Autodesk Inventor part; units mm, degrees
ref_plane "YZ Plane" through (0, 0, 0) normal (1, 0, 0) x (0, 1, 0)
ref_plane "XZ Plane" through (0, 0, 0) normal (0, 1, 0) x (-1, 0, 0)
ref_plane "XY Plane" through (0, 0, 0) normal (0, 0, 1) x (1, 0, 0)
sketch "main" plane through (0, 0, 0) normal (0, 0, 1) x (1, 0, 0)
  circle A0 centre (11.2296, 26.3602) radius 2.1844
  line L0 (23.9296, 20.0102) -> (22.6596, 20.0102)
  line L1 (4.8796, 31.6942) -> (5.8956, 32.7102)
  circle A1 centre (23.9296, 26.3602) radius 2.1844
  line L2 (23.9296, 32.7102) -> (5.8956, 32.7102)
  arc A2 (23.9296, 20.0102) -> (23.9296, 32.7102) centre (23.9296, 26.3602) ccw
  circle A3 centre (-14.1704, -24.4398) radius 2.1844
  circle A4 centre (11.2296, -24.4398) radius 2.1844
  arc A5 (22.6596, 20.0102) -> (4.8796, 2.2302) centre (22.6596, 2.2302) ccw
  line L3 (4.8796, -11.7398) -> (4.8796, 2.2302)
  arc A6 (4.8796, -11.7398) -> (11.2296, -18.0898) centre (11.2296, -11.7398) ccw
  line L4 (4.8796, 31.6942) -> (-20.5204, -19.1058)
  arc A7 (11.2296, -30.7898) -> (11.2296, -18.0898) centre (11.2296, -24.4398) ccw
  line L5 (11.2296, -30.7898) -> (-14.1704, -30.7898)
  line L6 (-20.5204, -24.4398) -> (-20.5204, -19.1058)
  arc A8 (-20.5204, -24.4398) -> (-14.1704, -30.7898) centre (-14.1704, -24.4398) ccw
  circle A9 centre (-4.1968, 2.8922) radius 2.0955
  point P0 (6.0044, -0.2269)
  dimension "d0" = 12.7
  dimension "d1" = 17.78
  dimension "d2" = 6.35
  dimension "d3" = 1.27
  dimension "d4" = 6.35
  dimension "d8" = 4.191
sketch "Sketch1" plane through (0, 0, 0) normal (0, 1, 0) x (-1, 0, 0)
  circle A0 centre (-12.7, 0) radius 2.1844
  line L0 (0, -6.35) -> (-1.27, -6.35)
  line L1 (-19.05, 5.334) -> (-18.034, 6.35)
  circle A1 centre (0, 0) radius 2.1844
  line L2 (0, 6.35) -> (-18.034, 6.35)
  arc A2 (0, -6.35) -> (0, 6.35) centre (0, 0) ccw
  circle A3 centre (-38.1, -50.8) radius 2.1844
  circle A4 centre (-12.7, -50.8) radius 2.1844
  arc A5 (-1.27, -6.35) -> (-19.05, -24.13) centre (-1.27, -24.13) ccw
  line L3 (-19.05, -38.1) -> (-19.05, -24.13)
  arc A6 (-19.05, -38.1) -> (-12.7, -44.45) centre (-12.7, -38.1) ccw
  line L4 (-19.05, 5.334) -> (-44.45, -45.466)
  arc A7 (-12.7, -57.15) -> (-12.7, -44.45) centre (-12.7, -50.8) ccw
  line L5 (-12.7, -57.15) -> (-38.1, -57.15)
  line L6 (-44.45, -50.8) -> (-44.45, -45.466)
  arc A8 (-44.45, -50.8) -> (-38.1, -57.15) centre (-38.1, -50.8) ccw
  circle A9 centre (-28.1264, -23.468) radius 2.0955
extrude "Extrusion1" add sketch "Sketch1" along normal blind 1.5875
properties part number "Front Gusset" material "Acetal Resin, White"
Model file for the job. Use its own axes, mm. A direction names the side the tool comes from. Give positions to 0.01 mm unless a question says otherwise; leave off trailing zeros. Order: outer loops, then holes, each group sorted by start corner. A loop starts at its lowest first (then second) coordinate and runs counter-clockwise, first axis right, second up. Notation, with made-up numbers: (50.5, 75) - (104.5, 75) arc R16 cw to (104.5, 93) - close; hole circle Ø6 at (25, 46). An arc over 180 degrees is marked (long way). Write item = value, one per line. Start each with the question number.
1. Cut at D-D, the plane z = -42.5. List the corners of the cut face in (x, y), and give its area (3 significant figures).
2. Drop flat-ended pins along their axis: P1, Ø0.5, axis at y = 0.5, z = -29, coming from the -X side; P2, Ø2.5, axis at x = 0, z = 0, coming from the -Y side. Give the stop position or say it passes through.
3. Cut at A-A, the plane z = 0. List the corners of the cut face in (x, y), and give its area (3 significant figures).
4. Which spindle directions (+Z, -Z, +X, -X, +Y, -Y) get a long thin tool onto all of the face, cutting with end or side? Do faces 5 (the flat face through (19.05, 1, -31)), 6 (the cylindrical face through (39.71, 0.783, -52.276)), 7 (the flat face through (1, 1, -6.35)). Say none if no direction does.
5. Probe line 1 along Z through (x, y) = (0, 1.1); line 2 along Z through (x, y) = (12.7, 1.15); line 3 along Z through (x, y) = (17, 1.35). List the from-to ranges inside material, lowest first.
6. Two-plate mould, pull along Z, no slides. Class faces 1 (the cylindrical face through (13.98, 0.783, -11.697)), 2 (the flat face through (31.57, 0.78, -19.71)), 3 (the flat face through (25, 1, -57.15)), 4 (the flat face through (19.4, 1.588, -25)): pulls with the +Z half, pulls with the -Z half, needs draft (parallel to the pull), parting line crosses it, or undercut.
7. Cut at C-C, the plane x = 41. List the corners of the cut face in (y, z), and give its area (3 significant figures).
8. Cut at B-B, the plane y = 0.75. List the corners of the cut face in (x, z), and give its area (3 significant figures).
Taken from the geometry:
q1.outline = (17.28, 0) - (42.97, 0) - (42.97, 1.59) - (17.28, 1.59) - close
q1.area = 40.8 mm²
q2.P1 = 19.05
q2.P2 = through
q3.outline = (-6.35, 0) - (-2.18, 0) - (-2.18, 1.59) - (-6.35, 1.59) - close; (2.18, 0) - (10.52, 0) - (10.52, 1.59) - (2.18, 1.59) - close; (14.88, 0) - (21.72, 0) - (21.72, 1.59) - (14.88, 1.59) - close
q3.area = 30.7 mm²
q4.face_5 = -X, +Y, -Y
q4.face_6 = +Y, -Y
q4.face_7 = -Z, -X, +Y, -Y
q5.line_1 = -6.35 to -2.18, 2.18 to 6.35
q5.line_2 = -57.15 to -52.98, -48.62 to -44.45, -10.51 to -2.18, 2.18 to 6.35
q5.line_3 = -57.15 to -42.77, -15.84 to 6.35
q6.face_1 = undercut
q6.face_2 = pulls with the +Z half
q6.face_3 = pulls with the -Z half
q6.face_4 = needs draft
q7.outline = (0, -56.45) - (1.59, -56.45) - (1.59, -38.57) - (0, -38.57) - close
q7.area = 28.4 mm²
q8.outline = (0, -6.35) - (1.27, -6.35) arc R17.78 cw to (19.05, -24.13) - (19.05, -38.1) arc R6.35 cw to (12.7, -44.45) arc R6.35 ccw to (12.7, -57.15) - (38.1, -57.15) arc R6.35 ccw to (44.45, -50.8) - (44.45, -45.47) - (19.05, 5.33) - (18.03, 6.35) - (0, 6.35) arc R6.35 ccw to start; hole circle Ø4.37 at (0, 0); hole circle Ø4.37 at (12.7, -50.8); hole circle Ø4.37 at (12.7, 0); hole circle Ø4.19 at (28.13, -23.47); hole circle Ø4.37 at (38.1, -50.8)
q8.area = 1,380 mm²
